Autodesk Inventor part; units mm, degrees
ref_plane "YZ Plane" through (0, 0, 0) normal (1, 0, 0) x (0, 1, 0)
ref_plane "XZ Plane" through (0, 0, 0) normal (0, 1, 0) x (-1, 0, 0)
ref_plane "XY Plane" through (0, 0, 0) normal (0, 0, 1) x (1, 0, 0)
sketch "Sketch1" plane through (0, 0, 0) normal (0, 1, 0) x (-1, 0, 0)
  line L0 (0, 0) -> (18.415, 0)
  line L1 (18.415, 0) -> (18.415, -19.05)
  line L2 (18.415, -19.05) -> (0, -19.05)
  line L3 (0, 0) -> (0, 5.08)
  line L4 (6.35, 5.08) -> (23.495, 5.08)
  line L5 (23.495, 5.08) -> (23.495, -24.13)
  line L6 (23.495, -24.13) -> (6.35, -24.13)
  line L7 (0, -23.495) -> (0, -19.05)
  line L8 (0, 5.08) -> (0, 24.13)
  line L9 (0, 24.13) -> (6.35, 24.13)
  line L10 (6.35, 24.13) -> (6.35, 5.08)
  line L11 (0, -23.495) -> (0, -43.18)
  line L12 (0, -43.18) -> (6.35, -43.18)
  line L13 (6.35, -43.18) -> (6.35, -24.13)
  dimension "d2" = 18.415
  dimension "d3" = 19.05
  dimension "d4" = 18.415
  dimension "d5" = 5.08
  dimension "d6" = 5.08
  dimension "d7" = 5.08
  dimension "d8" = 6.35
  dimension "d9" = 6.35
  dimension "d10" = 24.13
  dimension "d11" = 24.13
extrude "Extrusion1" add sketch "Sketch1" along normal blind 25.4
fillet "Fillet1" radius 4.7625 1 edges at (-18.415, 12.7, 0)
fillet "Fillet2" radius 4.7625 1 edges at (-18.415, 12.7, -19.05)
fillet "Fillet3" radius 4.7625 1 edges at (-6.35, 12.7, 5.08)
fillet "Fillet4" radius 4.7625 1 edges at (-6.35, 12.7, -24.13)
fillet "Fillet5" radius 5.08 2 edges at (-23.495, 12.7, 5.08) (-23.495, 12.7, -24.13)
sketch "Sketch3" plane through (-6.35, 0, 24.13) normal (-1, 0, 0) x (0, 0, 1)
  circle A0 centre (-7.1501, 12.7) radius 1.905
  line L0 (-14.2875, 0) -> (0, 0)
  line L1 (0, 0) -> (0, 25.4)
  point P0 (-24.13, 0)
  dimension "d31" = 3.81
  dimension "d32" = 12.7
  dimension "d33" = 7.1501
extrude "Extrusion2" cut sketch "Sketch3" against normal up to surface (6.35 mm away)
sketch "Sketch4" plane through (-6.35, 0, -43.18) normal (-1, 0, 0) x (0, 0, 1)
  circle A0 centre (7.1501, 12.7) radius 1.905
  line L0 (0, 0) -> (14.2875, 0)
  line L1 (0, 0) -> (0, 25.4)
  point P0 (43.18, 0)
  dimension "d36" = 3.81
  dimension "d37" = 12.7
  dimension "d38" = 7.1501
extrude "Extrusion3" cut sketch "Sketch4" against normal up to surface (6.35 mm away)
properties part number "TubeHolderV1"
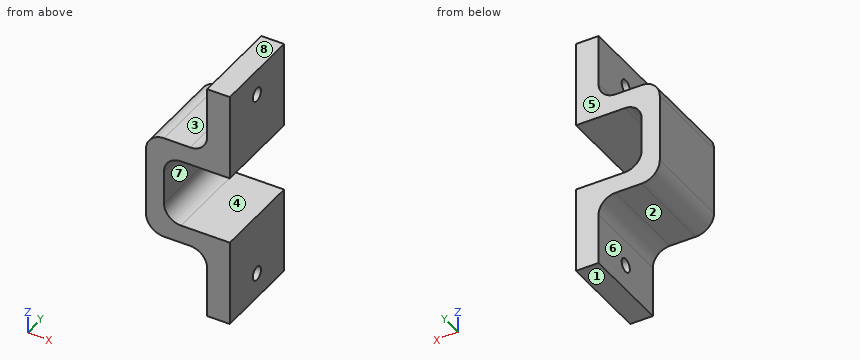
Check sheet for the modelled part. Datum: model origin and axes. Units: mm. Face numbers are marked on the shaded views. A direction names the side the tool comes from. Coordinates: 2 decimals unless noted, no trailing zeros. Write each loop counter-clockwise with the first axis right and the second up, starting at its lowest first coordinate (ties: lowest second). Pieces come first, ordered by that corner, then holes. Notation, with made-up numbers: (84.5, 23) -> (109.5, 23) arc R24 ccw to (109.5, 41) -> close; hole circle Ø8 at (78.5, 54). An arc over 180 degrees is marked (long way). Use a Markdown table: item, result.
1. Sectioned sample at A-A (x = -1.75). Enter the section's corners in (y, z) (3 decimals), plus the area to 3 significant figures.
Reported:
| item | result |
|---|---|
| outline | (0, -43.18) -> (25.4, -43.18) -> (25.4, -19.05) -> (0, -19.05) -> close; (0, 0) -> (25.4, 0) -> (25.4, 24.13) -> (0, 24.13) -> close; hole circle Ø3.81 at (12.7, -36.03); hole circle Ø3.81 at (12.7, 16.98) |
| area | 1,200 mm2 |
2. Sectioned sample at B-B (y = 12.7). Give the number of separate pieces and of enclosed holes in the cut face, plus the area to 3 significant figures.
Reported:
| item | result |
|---|---|
| separate pieces | 3 |
| enclosed holes | 0 |
| area | 537 mm2 |
3. Scan lines: line 1 along Z through (x, y) = (-11.75, 8.5); line 2 along Z through (x, y) = (-6.25, 8.25); line 3 along X through (y, z) = (18.5, 16). Record each from-to range of solid material in increasing order.
Reported:
| item | result |
|---|---|
| line 1 | z = -24.13 to -19.05, 0 to 5.08 |
| line 2 | z = -43.18 to -19.05, 0 to 24.13 |
| line 3 | x = -6.35 to 0 |
4. Sectioned sample at C-C (x = -17). Enter the section's corners in (y, z), plus the area to 3 significant figures.
Reported:
| item | result |
|---|---|
| outline | (0, -24.13) -> (25.4, -24.13) -> (25.4, -17.68) -> (0, -17.68) -> close; (0, -1.37) -> (25.4, -1.37) -> (25.4, 5.08) -> (0, 5.08) -> close |
| area | 328 mm2 |
5. Go/stop test with flat-tipped pins: pin 1 Ø8 at (y, z) = (14.5, -2) entering from +X; pin 2 Ø4 at (x, y) = (-13.5, 18) entering from -Z; pin 3 Ø1.5 at (y, z) = (15, -32.5) entering from -X; pin 4 Ø3.5 at (x, y) = (-14.5, 15) entering from +Z. Record where each tip stops, or that it passes through.
Reported:
| item | result |
|---|---|
| pin 1 | stops at x = 0 |
| pin 2 | stops at z = -24.13 |
| pin 3 | stops at x = -6.35 |
| pin 4 | stops at z = 5.08 |
6. Release check for a two-part mould opening along Z. For the marked faces 6, 7 and 8 record: pulls with the +Z half, pulls with the -Z half, needs draft (parallel to the pull), parting line crosses it, or undercut.
Reported:
| item | result |
|---|---|
| face 6 | needs draft |
| face 7 | undercut |
| face 8 | pulls with the +Z half |
7. Tool access check on the marked faces 1, 2, 3, 4 and 5. Record the directions out of +Z, -Z, +X, -X, +Y, -Y that give a thin tool (end or side, any length) a straight path to the whole face; none if there is none.
Reported:
| item | result |
|---|---|
| face 1 | -Z, +X, -X, +Y, -Y |
| face 2 | -Z, -X, +Y, -Y |
| face 3 | +Z, -X, +Y, -Y |
| face 4 | +X, +Y, -Y |
| face 5 | +Z, -Z, +X, -X, +Y |
